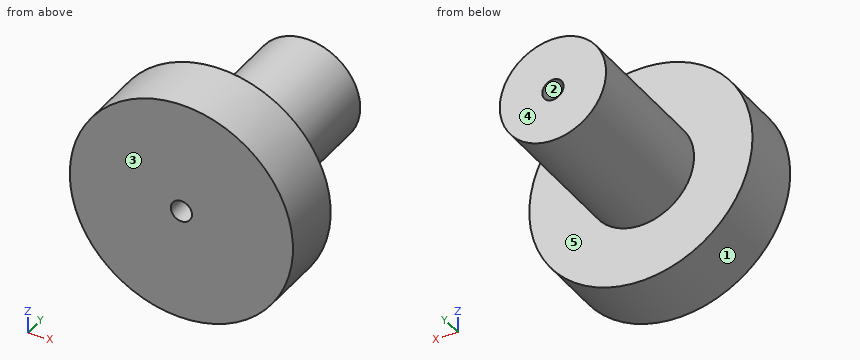
Autodesk Inventor part; units mm, degrees
ref_plane "YZ Plane" through (0, 0, 0) normal (1, 0, 0) x (0, 1, 0)
ref_plane "XZ Plane" through (0, 0, 0) normal (0, 1, 0) x (-1, 0, 0)
ref_plane "XY Plane" through (0, 0, 0) normal (0, 0, 1) x (1, 0, 0)
sketch "スケッチ1" plane through (0, 0, 0) normal (0, 1, 0) x (-1, 0, 0)
  circle A0 centre (0, 0) radius 5.25
  dimension "d0" = 10.5
extrude "押し出し1" add sketch "スケッチ1" along normal blind 3
sketch "スケッチ2" plane through (0, 3, 0) normal (0, 1, 0) x (1, 0, 0)
  circle A0 centre (0, 0) radius 2.5
  dimension "d3" = 5
extrude "押し出し2" add sketch "スケッチ2" along normal blind 7
sketch "スケッチ3" plane through (0, 10, 0) normal (0, 1, 0) x (1, 0, 0)
  circle A0 centre (0, 0) radius 2.5
  circle A1 centre (0, 0) radius 0.5
  dimension "d6" = 1
extrude "押し出し3" cut sketch "スケッチ3" against normal through all contours A1
properties part number "gear_tamiya_m0.5_10T_21T"
Work out the finished part from the listing and answer in its coordinate system (mm). Face numbers are marked on the shaded views. A direction names the side the tool comes from. Give positions to 0.01 mm unless a question says otherwise; leave off trailing zeros. Write each loop counter-clockwise with the first axis right and the second up, starting at its lowest first coordinate (ties: lowest second). Pieces come first, ordered by that corner, then holes. Notation, with made-up numbers: (47.25, 42) -> (85.25, 42) arc R20 ccw to (85.25, 49) -> close; hole circle Ø1 at (75.25, 17). An arc over 180 degrees is marked (long way). Write item = value, one per line.
Q1. For a pull along X with two mould halves and no side action, classify the marked faces 1, 2 and 3 as pulls with the +X half, pulls with the -X half, needs draft (parallel to the pull), parting line crosses it, or undercut.
Computed values:
face_1 = parting line crosses it
face_2 = undercut
face_3 = needs draft
Q2. Section B-B on z = 0 is taken. Determine the outline of the cut face in (x, y).
Computed values:
outline = (-5.25, 0) -> (-0.5, 0) -> (-0.5, 10) -> (-2.5, 10) -> (-2.5, 3) -> (-5.25, 3) -> close; (0.5, 0) -> (5.25, 0) -> (5.25, 3) -> (2.5, 3) -> (2.5, 10) -> (0.5, 10) -> close
Q3. Flat-ended cylindrical pins translate along their axes: pin 1 Ø4 at (y, z) = (8.5, -2) entering from +X; pin 2 Ø6 at (x, y) = (2, 7) entering from -Z; pin 3 Ø1.5 at (x, y) = (1, 3) entering from -Z. Find the tip coordinate at first contact, or state that the pin passes through.
Computed values:
pin_1 = 2.5
pin_2 = -2.5
pin_3 = -5.24
Q4. A tool of negligible diameter and unlimited length cuts with its end or side. For the marked faces 4 and 5, from which of +Z, -Z, +X, -X, +Y, -Y can it reach the whole face along a straight path? Write none if from no direction.
Computed values:
face_4 = +Z, -Z, +X, -X, +Y
face_5 = +Y
Q5. Section A-A on x = 0 is taken. Determine the outline of the cut face in (y, z), and give its area (3 significant figures).
Computed values:
outline = (0, -5.25) -> (3, -5.25) -> (3, -2.5) -> (10, -2.5) -> (10, -0.5) -> (0, -0.5) -> close; (0, 0.5) -> (10, 0.5) -> (10, 2.5) -> (3, 2.5) -> (3, 5.25) -> (0, 5.25) -> close
area = 56.5 mm^2
Q6. Section C-C on y = 2.75 is taken. Determine the outline of the cut face in (x, z).
Computed values:
outline = circle Ø10.5 at (0, 0); hole circle Ø1 at (0, 0)
Q7. Section D-D on x = -4.25 is taken. Determine the outline of the cut face in (y, z), and give its area (3 significant figures).
Computed values:
outline = (0, -3.08) -> (3, -3.08) -> (3, 3.08) -> (0, 3.08) -> close
area = 18.5 mm^2
Q8. Consider line 1 along Z through (x, y) = (0, 2.75); line 2 along X through (y, z) = (5, 0). Determine where each line is inside the solid, lowest interval first.
Computed values:
line_1 = -5.25 to -0.5, 0.5 to 5.25
line_2 = -2.5 to -0.5, 0.5 to 2.5
